CAD build for the part. Positions are in the model's coordinates, mm. A direction names the side the tool comes from. Give positions to 0.01 mm unless a question says otherwise; leave off trailing zeros. Write each loop counter-clockwise with the first axis right and the second up, starting at its lowest first coordinate (ties: lowest second). Pieces come first, ordered by that corner, then holes. Notation, with made-up numbers: (2, 70) - (22, 70) arc R21 ccw to (22, 87) - close; hole circle Ø7 at (85.25, -14). An arc over 180 degrees is marked (long way). Put each result on its own line as item: value. Start each with the question number.
1. Tool access for faces 4 (the cylindrical face through (10.71, 25.27, 20.14)), 5 (the flat face through (-10, 12, 35)), 6 (the flat face through (-10, 37, 35)): list every direction of +Z, -Z, +X, -X, +Y, -Y with a clear straight run to the whole face (end or side of a thin tool).
2. Wall check: line 1 (X direction, y = 25, z = 24.5); line 2 (X direction, y = 25, z = 36.25); line 3 (Z direction, x = -45.5, y = 36). Give the ranges that are in metal, low to high.
3. Cut at C-C on z = 12. List the corners of the cut face in (x, y), and give its area (3 significant figures).
4. Drop flat-ended pins along their axis: pin 1 (1 mm diameter, centred on x = -25, z = 34.5, fed in from +Y); pin 2 (5.5 mm diameter, centred on x = 0, y = 43, fed in from +Z); pin 3 (6 mm diameter, centred on y = 8.5, z = 32.5, fed in from -X). Give the stop position or say it passes through.
5. Cut at D-D on z = 7. List the corners of the cut face in (x, y), and give its area (3 significant figures).
6. Cut at B-B on x = 17. List the corners of the cut face in (y, z), and give its area (3 significant figures).
7. Mould opens along Y. For faces 1 (the flat face through (-20, 38, 35)), 2 (the cylindrical face through (-54.994, 24.45, 7.638)), 3 (the conical face through (-15.231, 25.211, 17.455)) say: +Y half, -Y half, draft (parallel to the pull), parting line (faces both ways), or undercut.
8. Cut at A-A on z = 24.5. List the corners of the cut face in (x, y), and give its area (3 significant figures).
from build123d import *

# Parameters (mm, degrees)
BOSS_EXTRUDE1_DEPTH            = 20
CUT_EXTRUDE10_DEPTH            = 10
CUT_EXTRUDE11_DEPTH            = 10
BOSS_EXTRUDE4_DEPTH            = 10
CUT_EXTRUDE16_DEPTH            = 20
BOSS_EXTRUDE6_DEPTH            = 10
SKETCH15_R                     = 2.5
CUT_EXTRUDE17_DEPTH            = 33
F_1_2_1_2_DIAMETER_HOLE2_D     = 10
F_1_2_1_2_DIAMETER_HOLE2_DEPTH = 20
F_1_2_1_2_DIAMETER_HOLE2_TIP   = 2.714778498


with BuildPart() as part:
    # Sketch1 → Boss-Extrude1 (new body)
    with BuildSketch(Plane.XY):
        with BuildLine():
            Line((-30, 50), (0, 50))
            ThreePointArc((0, 50), (25, 25), (0, 0))
            Line((0, 0), (-30, 0))
            ThreePointArc((-30, 0), (-55, 25), (-30, 50))
        make_face()
    extrude(amount=BOSS_EXTRUDE1_DEPTH)

    # Sketch2 → Cut-Extrude10 (cut)
    with BuildSketch(Plane.XY.offset(20)):
        with BuildLine():
            ThreePointArc((-47.853571071, 42.5), (-55, 25), (-47.853571071, 7.5))
            Line((-47.853571071, 7.5), (-47.853571071, 42.5))
        make_face()
    extrude(amount=-CUT_EXTRUDE10_DEPTH, mode=Mode.SUBTRACT)

    # Sketch9 → Cut-Extrude11 (cut)
    with BuildSketch(Plane.XY.offset(20)):
        with BuildLine():
            Line((17.853571071, 42.5), (17.853571071, 7.5))
            ThreePointArc((17.853571071, 7.5), (25, 25), (17.853571071, 42.5))
        make_face()
    extrude(amount=-CUT_EXTRUDE11_DEPTH, mode=Mode.SUBTRACT)

    # Sketch10 → Boss-Extrude4 (add)
    with BuildSketch(Plane.XY.offset(20)):
        with BuildLine():
            Line((-30, 45), (0, 45))
            ThreePointArc((0, 45), (20, 25), (0, 5))
            Line((0, 5), (-30, 5))
            ThreePointArc((-30, 5), (-50, 25), (-30, 45))
        make_face()
    extrude(amount=BOSS_EXTRUDE4_DEPTH)

    # Sketch11 → Cut-Extrude16 (cut)
    with BuildSketch(Plane.XY.offset(30)):
        with BuildLine():
            ThreePointArc((-47.853571071, 42.5), (-40.707142143, 25), (-47.853571071, 7.5))
            ThreePointArc((-47.853571071, 7.5), (-55, 25), (-47.853571071, 42.5))
        make_face()
        with BuildLine():
            ThreePointArc((17.853571071, 42.5), (10.707142143, 25), (17.853571071, 7.5))
            ThreePointArc((17.853571071, 7.5), (25, 25), (17.853571071, 42.5))
        make_face()
    extrude(amount=-CUT_EXTRUDE16_DEPTH, mode=Mode.SUBTRACT)

    # Sketch14 → Boss-Extrude6 (add)
    with BuildSketch(Plane.XY.offset(30)):
        with BuildLine():
            Line((-20, 40), (-20, 35))
            Line((-20, 35), (-10, 35))
            Line((-10, 35), (-10, 40))
            ThreePointArc((-10, 40), (5, 25), (-10, 10))
            Line((-10, 10), (-10, 15))
            Line((-10, 15), (-20, 15))
            Line((-20, 15), (-20, 10))
            ThreePointArc((-20, 10), (-35, 25), (-20, 40))
        make_face()
    extrude(amount=BOSS_EXTRUDE6_DEPTH)

    # Sketch15 → Cut-Extrude17 (cut)
    with BuildSketch(Plane.XY.offset(10)):
        with Locations((17.853571071, 25)):
            Circle(SKETCH15_R)
        with Locations((-47.853571071, 25)):
            Circle(SKETCH15_R)
    extrude(amount=-CUT_EXTRUDE17_DEPTH, mode=Mode.SUBTRACT)

    # Ø1.2 (1.2) Diameter Hole2
    with Locations(Plane(origin=(-15, 25, 40), x_dir=(1, 0, 0), z_dir=(0, 0, 1))):
        with Locations((0, 0)):
            Hole(F_1_2_1_2_DIAMETER_HOLE2_D / 2, depth=F_1_2_1_2_DIAMETER_HOLE2_DEPTH)
            with Locations((0, 0, -(F_1_2_1_2_DIAMETER_HOLE2_DEPTH + F_1_2_1_2_DIAMETER_HOLE2_TIP / 2))):  # 123° drill point
                Cone(0, F_1_2_1_2_DIAMETER_HOLE2_D / 2, F_1_2_1_2_DIAMETER_HOLE2_TIP, mode=Mode.SUBTRACT)


solid = part.part
Report:
1. face 4: +Z, +X
1. face 5: +Z, -Y
1. face 6: +Z, +Y
2. line 1: x = -40.71 to -20, -10 to 10.71
2. line 2: x = -35 to -20, -10 to 5
2. line 3: z = 0 to 10
3. outline: (-47.85, 7.5) arc R25 ccw to (-30, 0) - (0, 0) arc R25 ccw to (17.85, 7.5) arc R25 cw to (17.85, 42.5) arc R25 ccw to (0, 50) - (-30, 50) arc R25 ccw to (-47.85, 42.5) arc R25 cw to start
3. area: 2,770 mm²
4. pin 1: stops at y = 39.31
4. pin 2: stops at z = 30
4. pin 3: stops at x = -43.41
5. outline: (-30, 0) - (0, 0) arc R25 ccw to (0, 50) - (-30, 50) arc R25 ccw to start; hole circle Ø5 at (-47.85, 25); hole circle Ø5 at (17.85, 25)
5. area: 3,420 mm²
6. outline: (6.67, 0) - (22.65, 0) - (22.65, 10) - (8.42, 10) - (8.42, 20) - (6.67, 20) - close; (27.35, 0) - (43.33, 0) - (43.33, 20) - (41.58, 20) - (41.58, 10) - (27.35, 10) - close
6. area: 355 mm²
7. face 1: draft
7. face 2: parting line
7. face 3: undercut
8. outline: (-44.7, 11.44) arc R20 ccw to (-30, 5) - (0, 5) arc R20 ccw to (14.7, 11.44) arc R25 cw to (14.7, 38.56) arc R20 ccw to (0, 45) - (-30, 45) arc R20 ccw to (-44.7, 38.56) arc R25 cw to start; hole circle Ø10 at (-15, 25)
8. area: 2,030 mm²
